```python
from build123d import *

# Parameters (mm, degrees)
SKETCH1_W           = 15
SKETCH1_H           = 140
SKETCH1_R           = 3.75
BOSS_EXTRUDE1_DEPTH = 5
FILLET1_R           = 8


with BuildPart() as part:
    # Sketch1 → Boss-Extrude1 (new body)
    with BuildSketch(Plane(origin=(0, 0, 0), x_dir=(0, 0, -1), z_dir=(1, 0, 0))):
        Rectangle(SKETCH1_W, SKETCH1_H)
        Circle(SKETCH1_R, mode=Mode.SUBTRACT)
        with Locations((0, 60)):
            Circle(SKETCH1_R, mode=Mode.SUBTRACT)
        with Locations((0, -60)):
            Circle(SKETCH1_R, mode=Mode.SUBTRACT)
    extrude(amount=BOSS_EXTRUDE1_DEPTH)

    # Fillet1
    # the kernel refuses this fillet: 8 mm, written as the material it takes off along each edge
    with BuildSketch(Plane(origin=(-20, -70, 7.5), x_dir=(0, 0, -1), z_dir=(1, 0, 0))) as fillet1_piece_1:
        with BuildLine():
            CenterArc((FILLET1_R, FILLET1_R), FILLET1_R, 180, 90)
            Line((0, FILLET1_R), (0, 0))
            Line((0, 0), (FILLET1_R, 0))
        make_face()
    extrude(amount=45, mode=Mode.SUBTRACT)
    with BuildSketch(Plane(origin=(-20, -70, -7.5), x_dir=(0, 0, 1), z_dir=(1, 0, 0)), Plane(origin=(-20, 70, -7.5), x_dir=(0, -1, 0), z_dir=(1, 0, 0)), Plane(origin=(-20, 70, 7.5), x_dir=(0, 0, -1), z_dir=(1, 0, 0))) as fillet1_piece_2:
        with BuildLine():
            CenterArc((FILLET1_R, -FILLET1_R), FILLET1_R, 90, 90)
            Line((0, -FILLET1_R), (0, 0))
            Line((0, 0), (FILLET1_R, 0))
        make_face()
    extrude(amount=45, mode=Mode.SUBTRACT)


solid = part.part
```
Can you work these out from the model? Positions are in its coordinate system, mm. Coordinates: 2 decimals unless noted, no trailing zeros. Order: outer loops, then holes, each group sorted by start corner. A loop starts at its lowest first (then second) coordinate and runs counter-clockwise, first axis right, second up. Notation, with made-up numbers: (67, -36.5) - (123, -36.5) arc R33 cw to (123, 2.5) - close; hole circle Ø1 at (60, 88.25). An arc over 180 degrees is marked (long way). Answer in a Markdown table with one row per item.
1. If we mould it in two halves opening along Z, with no side actions, what happens to faces 1 (the flat face through (2, -1, 7.5)), 2 (the flat face through (0, 1, 5)), 3 (the cylindrical face through (2.465, 56.673, -1.73)), 4 (the cylindrical face through (2.46, -67.54, -5.27))? For each: pulls with the +Z half, pulls with the -Z half, needs draft (parallel to the pull), parting line crosses it, or undercut.
Reply:
| item | result |
|---|---|
| face 1 | pulls with the +Z half |
| face 2 | needs draft |
| face 3 | undercut |
| face 4 | pulls with the -Z half |
2. Suppose I cut it at B-B (x = 3.1). Please give me the cut outline in (y, z), and give its area (3 significant figures).
Reply:
| item | result |
|---|---|
| outline | (-69.98, 0) arc R8 ccw to (-62, -7.5) - (62, -7.5) arc R8 ccw to (69.98, 0) arc R8 ccw to (62, 7.5) - (-62, 7.5) arc R8 ccw to start; hole circle Ø7.5 at (-60, 0); hole circle Ø7.5 at (0, 0); hole circle Ø7.5 at (60, 0) |
| area | 1,910 mm^2 |
3. For pin 1 (1.5 mm diameter, centred on x = 1.5, z = 5.5, fed in from +Y), with a flat end and sliding along its axis, tell me the tip position at first contact or that it passes through.
Reply:
| item | result |
|---|---|
| pin 1 | stops at y = 68.04 |
4. Suppose I cut it at C-C (z = -5.5). Please give me the cut outline in (x, y), and give its area (3 significant figures).
Reply:
| item | result |
|---|---|
| outline | (0, -67.29) - (5, -67.29) - (5, 67.29) - (0, 67.29) - close |
| area | 673 mm^2 |
5. If I drill on line 1 along Y through (x, z) = (1.8, -0.25); line 2 along Y through (x, z) = (0.2, -1); line 3 along Y through (x, z) = (2.55, -5), over which ranges is the centre line in solid material (lowest first)?
Reply:
| item | result |
|---|---|
| line 1 | y = -69.96 to -63.74, -56.26 to -3.74, 3.74 to 56.26, 63.74 to 69.96 |
| line 2 | y = -69.86 to -63.61, -56.39 to -3.61, 3.61 to 56.39, 63.61 to 69.86 |
| line 3 | y = -67.81 to 67.81 |
6. Suppose I cut it at A-A (y = 0). Please give me the cut outline in (x, z).
Reply:
| item | result |
|---|---|
| outline | (0, -7.5) - (5, -7.5) - (5, -3.75) - (0, -3.75) - close; (0, 3.75) - (5, 3.75) - (5, 7.5) - (0, 7.5) - close |
